Verification items for the finished model (mm, model axes). Face numbers are marked on the shaded views. A direction names the side the tool comes from. Coordinates: 2 decimals unless noted, no trailing zeros. Order: outer loops, then holes, each group sorted by start corner. A loop starts at its lowest first (then second) coordinate and runs counter-clockwise, first axis right, second up. Notation, with made-up numbers: M -28,6.5 L 19,6.5 A28 cw 19,28.5 Z; hole C -35.5,33.5 d1. An arc over 180 degrees is marked long. Return JSON: item names as keys, results as strings.
```python
from build123d import *

# Parameters (mm, degrees)
F0_R     = 8.5
F0_R_2   = 5.5
F1_DEPTH = 1
F0_R_3   = 4.05
F2_DEPTH = 4.5
F0_R_4   = 3
F3_DEPTH = 7.5
F4_R     = 1
F5_R     = 1


with BuildPart() as f1:
    # F0 (on Front) → F1 (new body)
    with BuildSketch(Plane.XZ):
        Circle(F0_R)
        Circle(F0_R_2, mode=Mode.SUBTRACT)
    extrude(amount=F1_DEPTH)

    # F0 (on Front) → F2 (join)
    with BuildSketch(Plane.XZ):
        Circle(F0_R_2)
        Circle(F0_R_3, mode=Mode.SUBTRACT)
    extrude(amount=F2_DEPTH)

    # F0 (on Front) → F3 (join)
    with BuildSketch(Plane.XZ):
        Circle(F0_R_3)
        Circle(F0_R_4, mode=Mode.SUBTRACT)
    extrude(amount=F3_DEPTH)

    # F4
    f4_edges = [f1.edges().sort_by_distance(p)[0] for p in [
        (-3, -7.5, 0),
    ]]
    fillet(f4_edges, radius=F4_R)

    # F5
    f5_edges = [f1.edges().sort_by_distance(p)[0] for p in [
        (-3, 0, 0),
    ]]
    fillet(f5_edges, radius=F5_R)


solid = f1.part
```
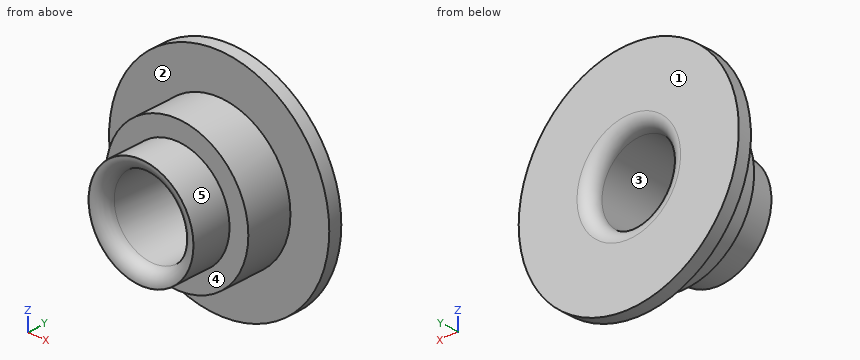
Q1. Cross-section at C-C, the plane y = -5.5. Record the boundary of the cut face in (x, z).
Values:
{"outline": "C 0,0 d8.1; hole C 0,0 d6"}
Q2. Cross-section at D-D, the plane z = -6. Record the boundary of the cut face in (x, y), and give its area (3 significant figures).
Values:
{"outline": "M -6.02,-1 L 6.02,-1 L 6.02,0 L -6.02,0 Z", "area": "12.0 mm^2"}
Q3. Material ranges on line 1 along Z through (x, y) = (0, -3.35); line 2 along Y through (x, z) = (4, -3.5); line 3 along Y through (x, z) = (-3, 6.75), recorded low to high.
Values:
{"line 1": "-5.5 to -3, 3 to 5.5", "line 2": "-4.5 to 0", "line 3": "-1 to 0"}
Q4. Go/stop test with flat-tipped pins: pin 1 (2 mm diameter, centred on y = -1.5, z = -4, fed in from -X); pin 2 (3 mm diameter, centred on x = 3, y = -5.5, fed in from +Z); pin 3 (3 mm diameter, centred on x = 2.5, y = -3, fed in from +Z); pin 4 (8 mm diameter, centred on x = 0, z = 0, fed in from +Y). Record where each tip stops, or that it passes through.
Values:
{"pin 1": "x = -7.9", "pin 2": "z = 5.17", "pin 3": "z = 5.41", "pin 4": "y = 0"}
Q5. Tool access check on the marked faces 1 and 2. Record the directions out of +Z, -Z, +X, -X, +Y, -Y that give a thin tool (end or side, any length) a straight path to the whole face; none if there is none.
Values:
{"face 1": "+Z, -Z, +X, -X, +Y", "face 2": "-Y"}
Q6. Draft check along X on the marked faces 3, 4 and 5. Enter one of: pulls with the +X half, pulls with the -X half, needs draft (parallel to the pull), parting line crosses it, or undercut.
Values:
{"face 3": "undercut", "face 4": "needs draft", "face 5": "parting line crosses it"}
Q7. Cross-section at A-A, the plane x = 0. Record the boundary of the cut face in (y, z), and give its area (3 significant figures).
Values:
{"outline": "M -7.5,-4.05 L -4.5,-4.05 L -4.5,-5.5 L -1,-5.5 L -1,-8.5 L 0,-8.5 L 0,-4 A1 ccw -1,-3 L -6.5,-3 A1 ccw -7.5,-4 Z; M -7.5,4 A1 ccw -6.5,3 L -1,3 A1 ccw 0,4 L 0,8.5 L -1,8.5 L -1,5.5 L -4.5,5.5 L -4.5,4.05 L -7.5,4.05 Z", "area": "33.9 mm^2"}
Q8. Cross-section at B-B, the plane z = 0. Record the boundary of the cut face in (x, y).
Values:
{"outline": "M -8.5,-1 L -5.5,-1 L -5.5,-4.5 L -4.05,-4.5 L -4.05,-7.5 L -4,-7.5 A1 ccw -3,-6.5 L -3,-1 A1 ccw -4,0 L -8.5,0 Z; M 3,-6.5 A1 ccw 4,-7.5 L 4.05,-7.5 L 4.05,-4.5 L 5.5,-4.5 L 5.5,-1 L 8.5,-1 L 8.5,0 L 4,0 A1 ccw 3,-1 Z"}
